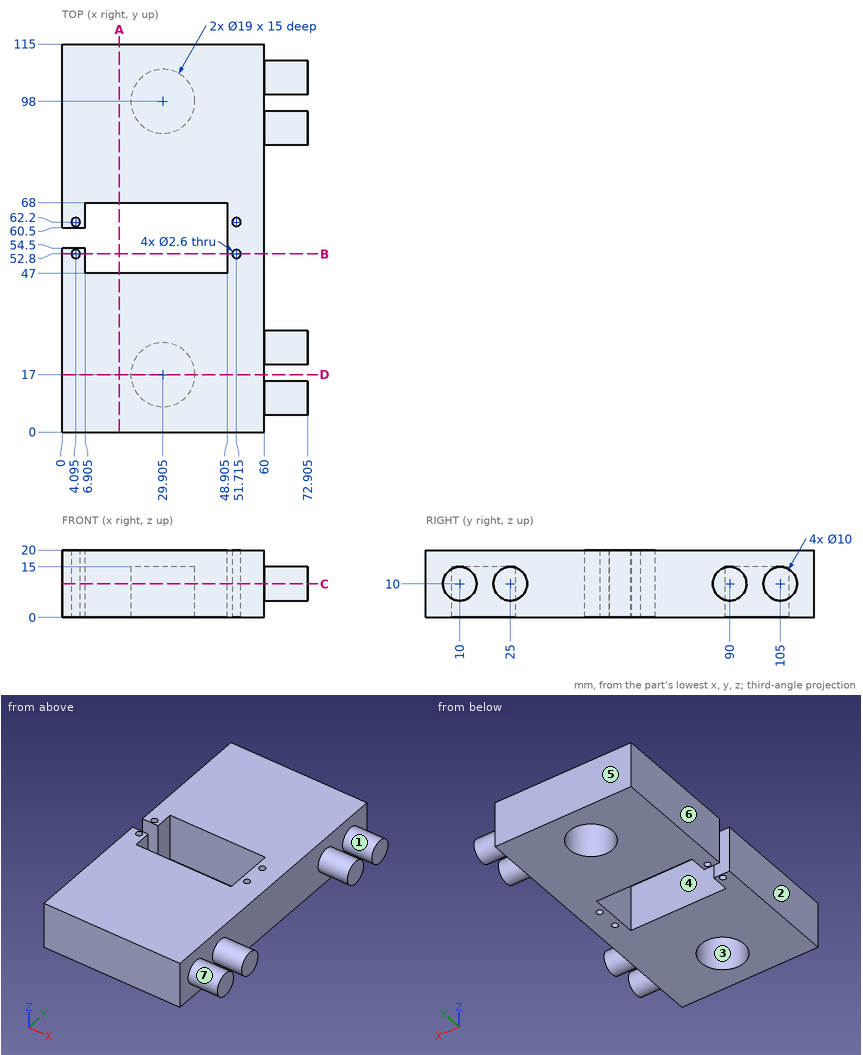
Design review of the part shown in the three views and the two pictorial views. Dimensions are in mm from the part's minimum x, y and z. A direction names the side the tool comes from. Give positions to 0.01 mm unless a question says otherwise; leave off trailing zeros. Loops run counter-clockwise (first coordinate to the right, second up) from the corner with the lowest first, then second, coordinate; pieces in that order, holes last. Notation, with made-up numbers: (67, 21.5) - (100, 21.5) arc R22 cw to (100, 40.5) - close; hole circle Ø9 at (-3, 67.25). An arc over 180 degrees is marked (long way). Use CSV: the item, a comma, the result in double quotes. Start each with the question number.
1. Draft analysis for pull direction Y (two halves, no side actions). For the marked faces 5, 6 and 7, state which applies: released by +Y, released by -Y, zero draft, split by the parting line, or undercut.
2. Insertion check: P1, Ø2, axis at y = 50.5, z = 5.5, coming from the +X side; P2, Ø3, axis at x = 63.5, y = 89.5, coming from the +Z side. Each pin has a flat end and moves straight along its axis. Give the tip position at first contact, or say it passes through.
3. Wall thickness on L1, parallel to X at y = 62, z = 8.5 (1 decimal); L2, parallel to Y at x = 15, z = 15.25; L3, parallel to Y at x = 61.5, z = 8: over which ranges is each line inside the solid? List them lowest first.
4. Add section B-B (y = 52.8). State the section outline as (x, z) points (1 decimal).
5. Add section D-D (y = 17). State the section outline as (x, z) points (1 decimal).
6. Machinability: for the marked faces 1, 2, 3 and 4, which of the approach directions +Z, -Z, +X, -X, +Y, -Y give a long, thin tool a straight path to every point of the face, cutting with its end or side? Answer none if there is none.
7. Add section A-A (x = 17). State the section outline as (y, z) points.
8. Add section C-C (z = 10). Count the separate pieces of the cut face and the enclosed holes in it, plus the area to 3 significant figures.
Results found:
1,face 5,"released by +Y"
1,face 6,"zero draft"
1,face 7,"undercut"
2,P1,"stops at x = 60"
2,P2,"stops at z = 15"
3,L1,"x = 0 to 2.8, 5.4 to 6.9, 48.9 to 50.4, 53 to 60"
3,L2,"y = 0 to 47, 68 to 115"
3,L3,"y = 5.42 to 14.58, 20.42 to 29.58, 85.42 to 94.58, 100.42 to 109.58"
4,outline,"(0, 0) - (2.8, 0) - (2.8, 20) - (0, 20) - close; (5.4, 0) - (6.9, 0) - (6.9, 20) - (5.4, 20) - close; (48.9, 0) - (50.4, 0) - (50.4, 20) - (48.9, 20) - close; (53, 0) - (60, 0) - (60, 20) - (53, 20) - close"
5,outline,"(0, 0) - (20.4, 0) - (20.4, 15) - (39.4, 15) - (39.4, 0) - (60, 0) - (60, 20) - (0, 20) - close"
6,face 1,"+X"
6,face 2,"+Z, -Z, -X, +Y, -Y"
6,face 3,"-Z"
6,face 4,"+Z, -Z"
7,outline,"(0, 0) - (47, 0) - (47, 20) - (0, 20) - close; (68, 0) - (115, 0) - (115, 20) - (68, 20) - close"
8,separate pieces,"1"
8,enclosed holes,"6"
8,area,"5,900 mm²"
